from build123d import *

# Parameters (mm, degrees)
SKETCH_8_R               = 16
EXTRUDE_3_DEPTH          = 20
SKETCH_8_4_R             = 20
EXTRUDE_4_DEPTH          = 40
CUT_EXTRUDE_6_REACH      = 120.709
CUT_EXTRUDE_7_DEPTH      = 110.963350072
CUT_EXTRUDE_7_DEPTH_BACK = 110.963350072
SKETCH_11_R              = 3.05
SKETCH_12_R              = 16.025
CUT_EXTRUDE_8_DEPTH      = 30
CUT_EXTRUDE_9_DEPTH      = 110.963350221
CUT_EXTRUDE_9_DEPTH_BACK = 110.963350221
SKETCH_14_R              = 3.05


with BuildPart() as part:
    # Sketch 8 → Extrude 3 (new body)
    with BuildSketch(Plane(origin=(0, 0, 0), x_dir=(1, 0, 0), z_dir=(0, 1, 0))):
        with Locations(Location((79.639435379, -3.747026688, 0), (0, 0, 270))):
            Circle(SKETCH_8_R)
    extrude(amount=EXTRUDE_3_DEPTH)

    # Sketch 8_4 → Extrude 4 (add)
    with BuildSketch(Plane(origin=(0, 0, 0), x_dir=(1, 0, 0), z_dir=(0, 1, 0))):
        with Locations(Location((79.639435379, -3.747026688, 0), (0, 0, 270))):
            Circle(SKETCH_8_4_R)
    extrude(amount=-EXTRUDE_4_DEPTH)

    # Sketch 10 → Cut-Extrude 6 (cut, up to next)
    with BuildSketch(Plane(origin=(0, 20, 0), x_dir=(1, 0, 0), z_dir=(0, 1, 0)), mode=Mode.PRIVATE) as cut_extrude_6_sk1:
        with BuildLine():
            Line((84.835587801, -0.747026688), (89.639435379, -0.747026688))
            Line((89.639435379, -0.747026688), (89.639435379, -6.747026688))
            Line((89.639435379, -6.747026688), (84.835587801, -6.747026688))
            ThreePointArc((84.835587801, -6.747026688), (79.639435379, -9.747026688), (74.443282956, -6.747026688))
            Line((74.443282956, -6.747026688), (69.639435379, -6.747026688))
            Line((69.639435379, -6.747026688), (69.639435379, -0.747026688))
            Line((69.639435379, -0.747026688), (74.443282956, -0.747026688))
            ThreePointArc((74.443282956, -0.747026688), (79.639435379, 2.252973312), (84.835587801, -0.747026688))
        make_face()
    cut_extrude_6_tool1 = extrude(cut_extrude_6_sk1.sketch, amount=-CUT_EXTRUDE_6_REACH, mode=Mode.PRIVATE) & part.part
    add(cut_extrude_6_tool1.solids().sort_by_distance((79.639435, 20, 3.747027))[0], mode=Mode.SUBTRACT)

    # Sketch 11 → Cut-Extrude 7 (cut, two sides: drawn at the far end of the back side and taken through both)
    with BuildSketch(Plane.XY.offset(-CUT_EXTRUDE_7_DEPTH_BACK)):
        with Locations((79.639435379, -22)):
            Circle(SKETCH_11_R)
    extrude(amount=CUT_EXTRUDE_7_DEPTH + CUT_EXTRUDE_7_DEPTH_BACK, mode=Mode.SUBTRACT)

    # Sketch 12 → Cut-Extrude 8 (cut)
    with BuildSketch(Plane.XZ.offset(40)):
        with Locations(Location((79.639435379, 3.747026688, 0), (0, 0, 270))):
            Circle(SKETCH_12_R)
    extrude(amount=-CUT_EXTRUDE_8_DEPTH, mode=Mode.SUBTRACT)

    # Sketch 14 → Cut-Extrude 9 (cut, two sides: drawn at the far end of the back side and taken through both)
    with BuildSketch(Plane.YZ.offset(-CUT_EXTRUDE_9_DEPTH_BACK)):
        with Locations(Location((-28, 3.747026688, 0), (0, 0, 90))):
            Circle(SKETCH_14_R)
    extrude(amount=CUT_EXTRUDE_9_DEPTH + CUT_EXTRUDE_9_DEPTH_BACK, mode=Mode.SUBTRACT)


solid = part.part
The model under review builds one solid part; all positions refer to its coordinate system, in mm. A direction names the side the tool comes from. Round coordinates to 2 decimals unless told otherwise and drop trailing zeros. Loops run counter-clockwise (first coordinate to the right, second up) from the corner with the lowest first, then second, coordinate; pieces in that order, holes last. Notation, with made-up numbers: M -35,13 L 7,13 A31 cw 7,39 Z; hole C 73,79 d4. An arc over 180 degrees is marked long. Answer as CSV lines item,"result". Start each with the question number.
Item 1: For faces 1 (the face through (93.1, 0, -5.2)), 2 (the face through (61.74, -25.29, 5.15)), 3 (the face through (80, -10, -3)), 4 (the face through (79.551, 5.21, -2.252)), list the 3-axis set-ups (+Z, -Z, +X, -X, +Y, -Y) from which the entire face can be reached by the end or side of a thin tool; tool diameter is ignored.
Item 2: Mouldability with a two-part tool opening along Z and no side actions: class faces 5 (the face through (76.592, -21.866, 21.583)), 6 (the face through (72, 5, 0.747)), 7 (the face through (71.979, -19.72, 22.222)) as released by +Z, released by -Z, zero draft, split by the parting line, or undercut.
Item 3: Consider section D-D (z = -5.5). Write out the cut boundary in (x, y), then the cut area to 3 significant figures.
Item 4: Consider section C-C (y = -22). Write out the cut boundary in (x, z) (3 decimals), then the cut area to 3 significant figures.
Item 5: Wall thickness on line 1 (Y direction, x = 66.5, z = 7); line 2 (Y direction, x = 73.5, z = -12.5); line 3 (Z direction, x = 82, y = 18): over which ranges is each line inside the solid? List them lowest first. Write a range as [from, to].
Item 6: Insertion check: P1, Ø4, axis at x = 86.5, y = 2.5, coming from the -Z side; P2, Ø3, axis at y = -27.5, z = -6, coming from the -X side; P3, Ø1.4, axis at x = 71.5, y = 3.5, coming from the -Z side. Each pin has a flat end and moves straight along its axis. Give the tip position at first contact, or say it passes through.
Item 7: Consider section B-B (z = 2). Write out the cut boundary in (x, y).
Item 8: Consider section A-A (x = 70.5). Write out the cut boundary in (y, z).
Answer:
1,face 1,"+Y"
1,face 2,"+X, -X"
1,face 3,"-Y"
1,face 4,"+Y, -Y"
2,face 5,"zero draft"
2,face 6,"undercut"
2,face 7,"split by the parting line"
3,outline,"M 61.91,-40 L 66.55,-40 L 66.55,-10 L 92.73,-10 L 92.73,-40 L 97.37,-40 L 97.37,0 L 92.7,0 L 92.7,20 L 66.58,20 L 66.58,0 L 61.91,0 Z"
3,area,"1,160 mm^2"
4,outline,"M 76.589,-16.019 L 76.589,-11.985 A16.025 cw 76.589,19.479 L 76.589,23.513 A20 ccw Z; M 82.689,-16.019 A20 ccw 82.689,23.513 L 82.689,19.479 A16.025 cw 82.689,-11.985 Z"
4,area,"401 mm^2"
5,line 1,"y = [-10, 20]"
5,line 2,"y = [-40, 0]"
5,line 3,"z = [-12.08, -1.77], [9.26, 19.57]"
6,P1,"stops at z = -11.5"
6,P2,"stops at x = 61.42"
6,P3,"stops at z = -10.42"
7,outline,"M 59.72,-40 L 63.71,-40 L 63.71,-30.5 L 59.72,-30.5 Z; M 59.72,-25.5 L 63.71,-25.5 L 63.71,-10 L 69.64,-10 L 69.64,20 L 63.74,20 L 63.74,0 L 59.72,0 Z; M 89.64,-10 L 95.57,-10 L 95.57,-25.5 L 99.56,-25.5 L 99.56,0 L 95.54,0 L 95.54,20 L 89.64,20 Z; M 95.57,-40 L 99.56,-40 L 99.56,-30.5 L 95.57,-30.5 Z"
8,outline,"M -40,-14.04 L 0,-14.04 L 0,-9.39 L 20,-9.39 L 20,0.75 L -10,0.75 L -10,-9.42 L -40,-9.42 Z; M -40,16.91 L -10,16.91 L -10,6.75 L 20,6.75 L 20,16.88 L 0,16.88 L 0,21.54 L -40,21.54 Z"
